Source: CAD feature listing. Evaluate the final solid. Frame: model axes, mm. A direction names the side the tool comes from. Coordinates: 2 decimals unless noted, no trailing zeros. Loops run counter-clockwise (first coordinate to the right, second up) from the corner with the lowest first, then second, coordinate; pieces in that order, holes last. Notation, with made-up numbers: (62.25, -2.5) -> (111.25, -2.5) arc R17 ccw to (111.25, 13.5) -> close; hole circle Ø11 at (38.5, -4.5). An arc over 180 degrees is marked (long way). Answer as a JSON object with one key per item and string values. Group by question number.
from build123d import *

# Parameters (mm, degrees)
F1_DEPTH = 69.85
F2_DEPTH = 69.85


with BuildPart() as f1:
    # F0 (on Front) → F1 (new body)
    with BuildSketch(Plane.XZ):
        Polygon((-132.521941, -100.065994), (-132.521941, -114.874194), (-56.321941, -114.874194), (99.58236, -11.216794), (70.170059, -11.216794), (49.088059, -11.216794), (49.088059, -26.024994), (28.006059, -26.024994), (28.006059, -40.833194), (6.924059, -40.833194), (6.924059, -55.641394), (-14.157941, -55.641394), (-14.157941, -70.449594), (-35.239941, -70.449594), (-35.239941, -85.257794), (-56.321941, -85.257794), (-56.321941, -100.065994), align=None)
        Polygon((70.170059, -11.216794), (99.58236, -11.216794), (146.370059, -11.216794), (146.370059, 3.591406), (70.170059, 3.591406), align=None)
    extrude(amount=F1_DEPTH)

    # F0 (on Front) → F2 (join)
    with BuildSketch(Plane.XZ):
        Polygon((-76.192113, 92.440606), (70.170059, -11.216794), (70.170059, 3.591406), (70.170059, 18.399606), (49.088059, 18.399606), (49.088059, 33.207806), (28.006059, 33.207806), (28.006059, 48.016006), (6.924059, 48.016006), (6.924059, 62.824206), (-14.157941, 62.824206), (-14.157941, 77.632406), (-35.239941, 77.632406), (-35.239941, 92.440606), (-56.321941, 92.440606), (-56.321941, 107.248806), (-132.521941, 107.248806), (-132.521941, 92.440606), align=None)
        Polygon((70.170059, -11.216794), (99.58236, -11.216794), (146.370059, -11.216794), (146.370059, 3.591406), (70.170059, 3.591406), align=None)
    extrude(amount=-F2_DEPTH)


solid = f1.part
1. Ray query, L1, parallel to Z at x = -78, y = 37; L2, parallel to Z at x = 134.5, y = 64; L3, parallel to X at y = 17.5, z = -6. Return the intervals inside material, ascending.
2. Pin query (flat end, axial travel): pin 1 Ø7.5 at (y, z) = (40, 59) entering from +X; pin 2 Ø10.5 at (x, y) = (-48.5, 38.5) entering from +Z; pin 3 Ø7.5 at (y, z) = (-52, -95.5) entering from -X; pin 4 Ø5 at (x, z) = (-10.5, 67) entering from -Y. Return the tip coordinate at first contact, or that it passes through.
3. Section query B-B on y = 42. Return loops of the section in (x, z), then the cut area to 3 significant figures.
4. Section query A-A on x = -43. Return loops of the section in (y, z).
5. Section query C-C on x = -3.5. Return loops of the section in (y, z).
6. Section query D-D on y = -54.5. Return loops of the section in (x, z) (3 decimals), then the cut area to 3 significant figures.
7. Reachability of faces 1 (the face through (70.17, -34, -4)), 2 (the face through (-25, 34, 77.632)), 3 (the face through (49.088, -34, -19)) from +Z, -Z, +X, -X, +Y, -Y: full face, straight path, thin tool, end or side. Return the list, or none.
Solved:
{
 "1": {"L1": "92.44 to 107.25", "L2": "-11.22 to 3.59", "L3": "62.8 to 146.37"},
 "2": {"pin 1": "x = 6.92", "pin 2": "z = 92.44", "pin 3": "x = -56.32", "pin 4": "through"},
 "3": {"outline": "(-132.52, 92.44) -> (-76.19, 92.44) -> (70.17, -11.22) -> (146.37, -11.22) -> (146.37, 3.59) -> (70.17, 3.59) -> (70.17, 18.4) -> (49.09, 18.4) -> (49.09, 33.21) -> (28.01, 33.21) -> (28.01, 48.02) -> (6.92, 48.02) -> (6.92, 62.82) -> (-14.16, 62.82) -> (-14.16, 77.63) -> (-35.24, 77.63) -> (-35.24, 92.44) -> (-56.32, 92.44) -> (-56.32, 107.25) -> (-132.52, 107.25) -> close", "area": "5,160 mm^2"},
 "4": {"outline": "(-69.85, -106.02) -> (0, -106.02) -> (0, -85.26) -> (-69.85, -85.26) -> close; (0, 68.93) -> (69.85, 68.93) -> (69.85, 92.44) -> (0, 92.44) -> close"},
 "5": {"outline": "(-69.85, -79.75) -> (0, -79.75) -> (0, -55.64) -> (-69.85, -55.64) -> close; (0, 40.96) -> (69.85, 40.96) -> (69.85, 62.82) -> (0, 62.82) -> close"},
 "6": {"outline": "(-132.522, -114.874) -> (-56.322, -114.874) -> (99.582, -11.217) -> (146.37, -11.217) -> (146.37, 3.591) -> (70.17, 3.591) -> (70.17, -11.217) -> (49.088, -11.217) -> (49.088, -26.025) -> (28.006, -26.025) -> (28.006, -40.833) -> (6.924, -40.833) -> (6.924, -55.641) -> (-14.158, -55.641) -> (-14.158, -70.45) -> (-35.24, -70.45) -> (-35.24, -85.258) -> (-56.322, -85.258) -> (-56.322, -100.066) -> (-132.522, -100.066) -> close", "area": "5,650 mm^2"},
 "7": {"face 1": "+Z, -X, -Y", "face 2": "+Z, +X, +Y, -Y", "face 3": "+Z, -X, +Y, -Y"}
}
